Verification items for the finished model (mm, model axes). Coordinates: 2 decimals unless noted, no trailing zeros. Loops run counter-clockwise (first coordinate to the right, second up) from the corner with the lowest first, then second, coordinate; pieces in that order, holes last.
Q1. Sectioned sample at A-A (z = 6.5). Enter the section's corners in (x, y), then the cut area to 3 significant figures.
Q2. Mould release check, pull along X, two halves, no side actions. Record for faces 1 (the face through (-27.128, 20.425, 0.21)), 2 (the face through (48, -14, -15)), 3 (the face through (-6, -8, 0)), 4 (the face through (52.47, 5.44, 0.21)): +X half, -X half, draft (parallel to the pull), parting line (faces both ways), or undercut.
Q3. Material ranges on probe 1 along Y at (x, z) = (-0.5, -12); probe 2 along Y at (x, z) = (106, -3.5); probe 3 along X at (y, z) = (-8, 3), recorded low to high.
Q4. Go/stop test with flat-tipped pins: P1, Ø8, axis at y = 15.5, z = -7, coming from the +X side; P2, Ø12, axis at x = -22, z = 9.5, coming from the -Y side; P3, Ø10, axis at x = 71.5, z = 1.5, coming from the -Y side. Record where each tip stops, or that it passes through.
Q5. Sectioned sample at B-B (y = -61). Enter the section's corners in (x, z), then the cut area to 3 significant figures.
Q6. Sectioned sample at C-C (x = -33). Enter the section's corners in (y, z), then the cut area to 3 significant figures.
```python
from build123d import *

# Parameters (mm, degrees)
EXTRUDE_1_DEPTH = 15


with BuildPart() as part:
    # 草图2 → 凸台-拉伸1 (new, symmetric)
    with BuildSketch(Plane.XY):
        with BuildLine():
            ThreePointArc((-50.101760938, 30.428374824), (-53.212480705, 35.199792857), (-48.662053388, 38.625667744))
            ThreePointArc((-48.662053388, 38.625667744), (53.783376909, 4.667316575), (132.921228365, -68.718215172))
            ThreePointArc((132.921228365, -68.718215172), (131.035363994, -82.914699935), (116.728010512, -82.285175988))
            ThreePointArc((116.728010512, -82.285175988), (65.281465021, -39.655460148), (6.814778353, -7.318387527))
            ThreePointArc((6.814778353, -7.318387527), (-5.74124488, -8.18768021), (-9.202597166, 3.913081318))
            ThreePointArc((-9.202597166, 3.913081318), (-27.419137904, 20.615137073), (-50.101760938, 30.428374824))
        make_face()
    extrude(amount=EXTRUDE_1_DEPTH, both=True)


solid = part.part
```
Geometry check:
1. outline: (-50.1, 30.43) arc R74.4 cw to (-9.2, 3.91) arc R10 ccw to (6.81, -7.32) arc R358.31 cw to (116.73, -82.29) arc R10.6 ccw to (132.92, -68.72) arc R254.32 ccw to (-48.66, 38.63) arc R4.17 ccw to start
1. area: 5,650 mm2
2. face 1: -X half
2. face 2: draft
2. face 3: undercut
2. face 4: +X half
3. probe 1: y = -9.99 to 28.71
3. probe 2: y = -71.99 to -36.25
3. probe 3: x = -6 to 6, 8.37 to 73.14
4. P1: stops at x = 41.46
4. P2: stops at y = 11.5
4. P3: stops at y = -47.63
5. outline: (93.48, -15) - (127.32, -15) - (127.32, 15) - (93.48, 15) - close
5. area: 1,020 mm2
6. outline: (23.9, -15) - (36.46, -15) - (36.46, 15) - (23.9, 15) - close
6. area: 377 mm2
